Check sheet for the modelled part. Datum: model origin and axes. Units: mm. Face numbers are marked on the shaded views. A direction names the side the tool comes from. Coordinates: 2 decimals unless noted, no trailing zeros. Loops run counter-clockwise (first coordinate to the right, second up) from the corner with the lowest first, then second, coordinate; pieces in that order, holes last. Notation, with made-up numbers: M -24.75,-0.5 L -3.75,-0.5 A10 cw -3.75,9.5 Z; hole C -17,54 d11. An arc over 180 degrees is marked long. Answer in a Markdown table with one row per item. Add a question column.
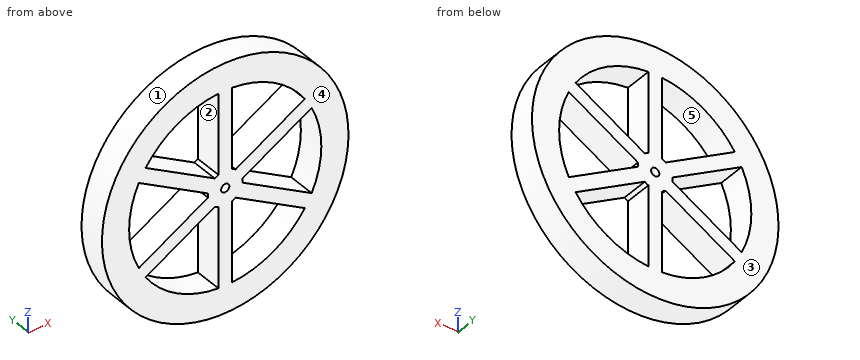
```python
from build123d import *

# Parameters (mm, degrees)
SKETCH1_R           = 45
SKETCH1_R_2         = 1.5
BOSS_EXTRUDE1_DEPTH = 10


with BuildPart() as part:
    # Sketch1 → Boss-Extrude1 (new body)
    with BuildSketch(Plane(origin=(0, 0, 0), x_dir=(1, 0, 0), z_dir=(0, 1, 0))):
        with Locations(Location((0, 0, 0), (0, 0, 270))):
            Circle(SKETCH1_R)
        with Locations(Location((0, 0, 0), (0, 0, 270))):
            Circle(SKETCH1_R_2, mode=Mode.SUBTRACT)
        with BuildLine():
            Line((-2.5, 5.837165408), (-2.5, 35))
            ThreePointArc((-2.5, 35), (-17.54458606, 30.388114453), (-29.060889132, 19.665063509))
            Line((-29.060889132, 19.665063509), (-3.805133529, 5.083646213))
            ThreePointArc((-3.805133529, 5.083646213), (-3.175, 5.499261314), (-2.5, 5.837165408))
        make_face(mode=Mode.SUBTRACT)
        with BuildLine():
            Line((2.5, 5.837165408), (2.5, 35))
            ThreePointArc((2.5, 35), (17.54458606, 30.388114453), (29.060889132, 19.665063509))
            Line((29.060889132, 19.665063509), (3.805133529, 5.083646213))
            ThreePointArc((3.805133529, 5.083646213), (3.175, 5.499261314), (2.5, 5.837165408))
        make_face(mode=Mode.SUBTRACT)
        with BuildLine():
            Line((6.305133529, 0.753519195), (31.560889132, 15.334936491))
            ThreePointArc((31.560889132, 15.334936491), (35.089172119, 0), (31.560889132, -15.334936491))
            Line((31.560889132, -15.334936491), (6.305133529, -0.753519195))
            ThreePointArc((6.305133529, -0.753519195), (6.35, 0), (6.305133529, 0.753519195))
        make_face(mode=Mode.SUBTRACT)
        with BuildLine():
            Line((3.805133529, -5.083646213), (29.060889132, -19.665063509))
            ThreePointArc((29.060889132, -19.665063509), (17.54458606, -30.388114453), (2.5, -35))
            Line((2.5, -35), (2.5, -5.837165408))
            ThreePointArc((2.5, -5.837165408), (3.175, -5.499261314), (3.805133529, -5.083646213))
        make_face(mode=Mode.SUBTRACT)
        with BuildLine():
            Line((-2.5, -5.837165408), (-2.5, -35))
            ThreePointArc((-2.5, -35), (-17.54458606, -30.388114453), (-29.060889132, -19.665063509))
            Line((-29.060889132, -19.665063509), (-3.805133529, -5.083646213))
            ThreePointArc((-3.805133529, -5.083646213), (-3.175, -5.499261314), (-2.5, -5.837165408))
        make_face(mode=Mode.SUBTRACT)
        with BuildLine():
            Line((-6.305133529, -0.753519195), (-31.560889132, -15.334936491))
            ThreePointArc((-31.560889132, -15.334936491), (-35.089172119, 0), (-31.560889132, 15.334936491))
            Line((-31.560889132, 15.334936491), (-6.305133529, 0.753519195))
            ThreePointArc((-6.305133529, 0.753519195), (-6.35, 0), (-6.305133529, -0.753519195))
        make_face(mode=Mode.SUBTRACT)
    extrude(amount=BOSS_EXTRUDE1_DEPTH)


solid = part.part
```
Q1. Access from +Z, -Z, +X, -X, +Y, -Y to the whole of each face (thin tool, end or side, straight path). Record for the marked faces 4 and 5.
Q2. Cross-section at D-D (x = 10.5). Record the cut outline in (y, z), plus the area to 3 significant figures.
Q3. Cross-section at B-B (y = 3.5). Record the cut outline in (x, z).
Q4. Mould release check, pull along X, two halves, no side actions. Record for the marked faces 1, 2 and 3: released by +X, released by -X, zero draft, split by the parting line, or undercut.
Q5. Go/stop test with flat-tipped pins: pin 1 (5 mm diameter, centred on y = 3, z = 6.5, fed in from -X); pin 2 (3 mm diameter, centred on x = 32.5, y = 6.5, fed in from +Z); pin 3 (4 mm diameter, centred on y = 3.5, z = 0, fed in from -X). Record where each tip stops, or that it passes through.
Q6. Cross-section at A-A (x = 0). Record the cut outline in (y, z).
Q7. Thickness scan on L1, parallel to X at y = 5.5, z = 0; L2, parallel to X at y = 2.75, z = 3.5; L3, parallel to X at y = 1, z = -6.5. Record the ranges inside material, lowest first.
Q8. Cross-section at C-C (z = -10.5). Record the cut outline in (x, y).
Answer key:
| question | item | result |
|---|---|---|
| 1 | face 4 | +Z, -Z, +X, -X, -Y |
| 1 | face 5 | +Y, -Y |
| 2 | outline | M 0,-43.76 L 10,-43.76 L 10,-33.48 L 0,-33.48 Z; M 0,-8.95 L 10,-8.95 L 10,-3.18 L 0,-3.18 Z; M 0,3.18 L 10,3.18 L 10,8.95 L 0,8.95 Z; M 0,33.48 L 10,33.48 L 10,43.76 L 0,43.76 Z |
| 2 | area | 321 mm^2 |
| 3 | outline | C 0,0 d90; hole M -31.56,-15.33 L -6.31,-0.75 A6.35 cw -6.31,0.75 L -31.56,15.33 A35.09 ccw Z; hole M -29.06,-19.67 A35.09 ccw -2.5,-35 L -2.5,-5.84 A6.35 cw -3.81,-5.08 Z; hole M -29.06,19.67 L -3.81,5.08 A6.35 cw -2.5,5.84 L -2.5,35 A35.09 ccw Z; hole C 0,0 d3; hole M 2.5,-35 A35.09 ccw 29.06,-19.67 L 3.81,-5.08 A6.35 cw 2.5,-5.84 Z; hole M 2.5,5.84 A6.35 cw 3.81,5.08 L 29.06,19.67 A35.09 ccw 2.5,35 Z; hole M 6.31,-0.75 L 31.56,-15.33 A35.09 ccw 31.56,15.33 L 6.31,0.75 A6.35 cw Z |
| 4 | face 1 | split by the parting line |
| 4 | face 2 | undercut |
| 4 | face 3 | zero draft |
| 5 | pin 1 | x = -44.82 |
| 5 | pin 2 | z = 32.62 |
| 5 | pin 3 | x = -45 |
| 6 | outline | M 0,-45 L 10,-45 L 10,-1.5 L 0,-1.5 Z; M 0,1.5 L 10,1.5 L 10,45 L 0,45 Z |
| 7 | L1 | -45 to -35.09, -6.35 to -1.5, 1.5 to 6.35, 35.09 to 45 |
| 7 | L2 | -44.86 to -34.91, -11.06 to 11.06, 34.91 to 44.86 |
| 7 | L3 | -44.53 to -34.48, -16.26 to -6.26, -2.5 to 2.5, 6.26 to 16.26, 34.48 to 44.53 |
| 8 | outline | M -43.76,0 L -33.48,0 L -33.48,10 L -43.76,10 Z; M -23.19,0 L -13.19,0 L -13.19,10 L -23.19,10 Z; M -2.5,0 L 2.5,0 L 2.5,10 L -2.5,10 Z; M 13.19,0 L 23.19,0 L 23.19,10 L 13.19,10 Z; M 33.48,0 L 43.76,0 L 43.76,10 L 33.48,10 Z |
